For this review, take the finished solid that the model builds, in its own axes (mm). A direction names the side the tool comes from. Coordinates: 2 decimals unless noted, no trailing zeros. Order: outer loops, then holes, each group sorted by start corner. A loop starts at its lowest first (then second) coordinate and runs counter-clockwise, first axis right, second up. Notation, with made-up numbers: (-33, 0.5) -> (-19, 0.5) arc R35 cw to (-19, 33.5) -> close; hole circle Ø1 at (-2.5, 37). An arc over 180 degrees is marked (long way). Answer as a JSON object with one key per item and string values. Group by question number.
1) Machinability: for faces 1 (the flat face through (0, -22, 44)), 2 (the flat face through (0, -27, 44)), 3 (the cylindrical face through (9.339, -24.535, 74.023)), which of the approach directions +Z, -Z, +X, -X, +Y, -Y give a long, thin tool a straight path to every point of the face, cutting with its end or side? Answer none if there is none.
2) Add section B-B, the plane y = 20. Write out the cut boundary in (x, z).
3) Add section A-A, the plane x = 0. Write out the cut boundary in (y, z), then the cut area to 3 significant figures.
4) For pin 1 (5 mm diameter, centred on x = -10, z = 57, fed in from -Y); pin 2 (1 mm diameter, centred on y = 23.5, z = 69, fed in from +X); pin 3 (2 mm diameter, centred on y = 24, z = 73, fed in from -X); pin 4 (10 mm diameter, centred on x = 12.5, y = 19.5, fed in from +Z), all flat-tipped, find the tip position at first contact; note any pin that passes through.
5) Add section D-D, the plane x = 8. Write out the cut boundary in (y, z).
6) Draft analysis for pull direction X (two halves, no side actions). For faces 4 (the flat face through (34, -14, 44)), 5 (the flat face through (0, -26, 90)), 6 (the cylindrical face through (-10.661, -24.535, 54.023)), state which applies: +X half, -X half, draft (parallel to the pull), parting line (faces both ways), or undercut.
7) Add section C-C, the plane z = 79. Write out the cut boundary in (x, y).
8) Wall thickness on L1, parallel to Z at x = -10, y = -25; L2, parallel to Y at x = -1, z = 24; L3, parallel to X at y = 0, z = 60.5: over which ranges is each line inside the solid? List them lowest first.
Autodesk Fusion 360 part; units mm, degrees
sketch "Sketch1" plane through (0, 0, 0) normal (0, 0, 1) x (1, 0, 0)
  circle A0 centre (0, 0) radius 30
  circle A1 centre (0, 0) radius 34
  line L0 (0, 30) -> (0, -22) construction
  line L1 (-20.3961, -22) -> (20.3961, -22)
  line L2 (-34, -27) -> (34, -27)
  line L3 (-34, -27) -> (-34, 0)
  line L4 (34, -27) -> (34, 0)
  circle A2 centre (0, 4) radius 25.4 construction
  dimension "d1" = 60
  dimension "d2" = 68
  dimension "d3" = 52
  dimension "d6" = 5
  dimension "d38" = 50.8
extrude "Extrude1" add sketch "Sketch1" along normal blind 90 contours A0 A1 L2 | A0 L1 L2 | A1 L2 L3 | A1 L2 L4 picked at (-32.5234, 2.2674)
sketch "Sketch8" plane through (0, -27, 0) normal (0, -1, 0) x (1, 0, 0)
  line L0 (-34, 0) -> (34, 0)
  line L1 (34, 0) -> (34, 90)
  line L2 (34, 90) -> (-34, 90)
  line L3 (-34, 90) -> (-34, 0)
  circle A0 centre (-10, 77) radius 3.05
  circle A1 centre (10, 77) radius 3.05
  circle A2 centre (-10, 57) radius 3.05
  circle A3 centre (10, 57) radius 3.05
  dimension "d43" = 6.1
  dimension "d44" = 6.1
  dimension "d45" = 6.1
  dimension "d46" = 6.1
  dimension "d47" = 13
  dimension "d48" = 13
  dimension "d49" = 33
  dimension "d50" = 33
  dimension "d51" = 20
  dimension "d52" = 20
  dimension "d53" = 24
  dimension "d54" = 24
extrude "Extrude10" cut sketch "Sketch8" against normal blind 5 contours A0 | A1 | A2 | A3
equation "d44 = d43"
equation "d45 = d43"
equation "d46 = d43"
equation "d48 = d47"
equation "d50 = d49"
equation "d52 = d51"
equation "d54 = d53"
Output values:
{
 "1": {"face 1": "+Z, -Z", "face 2": "+Z, -Z, +X, -X, -Y", "face 3": "-Y"},
 "2": {"outline": "(-27.5, 0) -> (-22.36, 0) -> (-22.36, 90) -> (-27.5, 90) -> close; (22.36, 0) -> (27.5, 0) -> (27.5, 90) -> (22.36, 90) -> close"},
 "3": {"outline": "(-27, 0) -> (-22, 0) -> (-22, 90) -> (-27, 90) -> close; (30, 0) -> (34, 0) -> (34, 90) -> (30, 90) -> close", "area": "810 mm²"},
 "4": {"pin 1": "stops at y = 27.27", "pin 2": "stops at x = 25.04", "pin 3": "stops at x = -25.04", "pin 4": "passes through"},
 "5": {"outline": "(-27, 0) -> (-22, 0) -> (-22, 54.7) -> (-27, 54.7) -> close; (-27, 59.3) -> (-22, 59.3) -> (-22, 74.7) -> (-27, 74.7) -> close; (-27, 79.3) -> (-22, 79.3) -> (-22, 90) -> (-27, 90) -> close; (28.91, 0) -> (33.05, 0) -> (33.05, 90) -> (28.91, 90) -> close"},
 "6": {"face 4": "+X half", "face 5": "draft", "face 6": "undercut"},
 "7": {"outline": "(-34, -27) -> (-12.3, -27) -> (-12.3, -22) -> (-20.4, -22) arc R30 cw (long way) to (20.4, -22) -> (12.3, -22) -> (12.3, -27) -> (34, -27) -> (34, 0) arc R34 ccw to (-34, 0) -> close; (-7.7, -27) -> (7.7, -27) -> (7.7, -22) -> (-7.7, -22) -> close"},
 "8": {"L1": "z = 0 to 53.95, 60.05 to 73.95, 80.05 to 90", "L2": "y = -27 to -22, 29.98 to 33.99", "L3": "x = -34 to -30, 30 to 34"}
}
